Geometry: see drawing. Coordinates: mm, zero at the bounding-box minimum. Give positions to 0.01 mm unless a question says otherwise; leave off trailing zeros. Order: outer loops, then holes, each group sorted by start corner. A loop starts at its lowest first (then second) coordinate and runs counter-clockwise, first axis right, second up. Notation, with made-up numbers: (55, 13) - (96, 13) arc R22 ccw to (96, 43) - close; hole circle Ø5 at (-24.5, 8.5). An arc over 180 degrees is marked (long way). One line per item, written item: value.
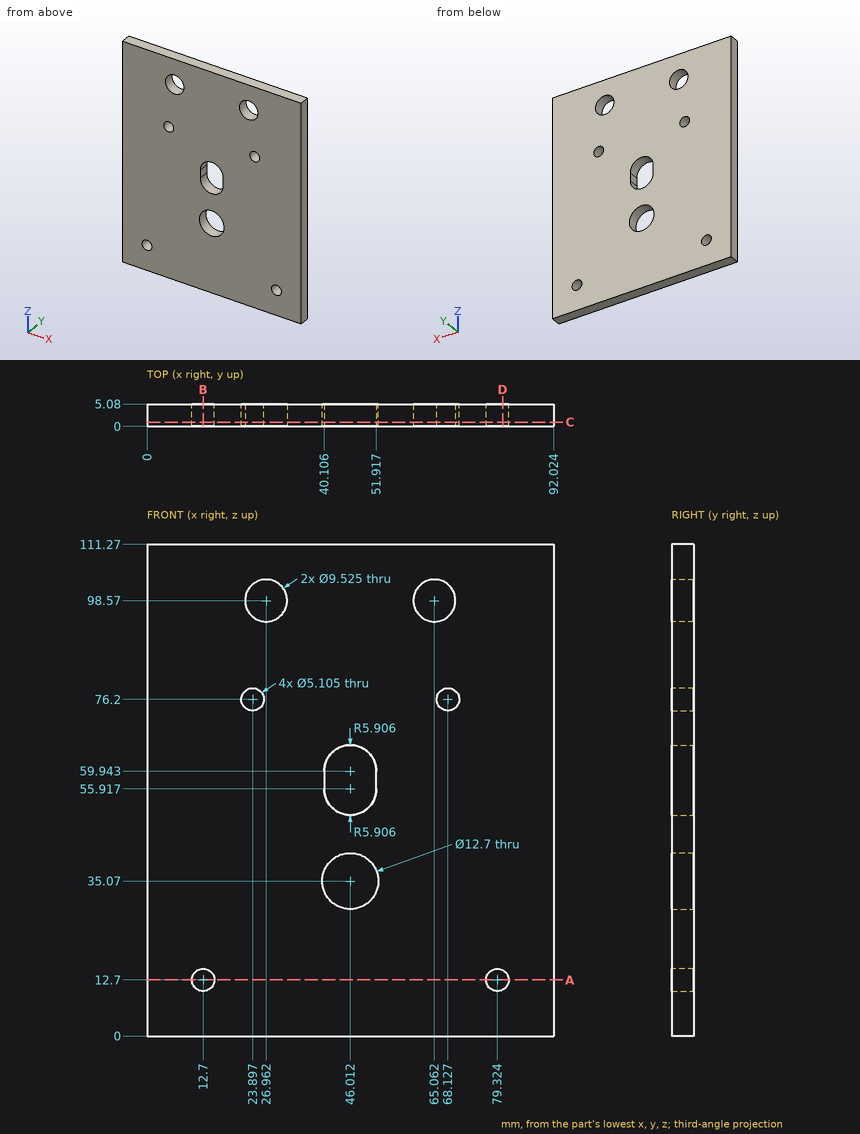
1) Section C-C, the plane y = 0.95. Count the separate pieces of the cut face and the enclosed holes in it, then the cut area to 3 significant figures.
Answers below:
separate pieces: 1
enclosed holes: 8
area: 9,730 mm^2
2) Section D-D, the plane x = 80.5. Return loops of the section in (y, z) (1 decimal), then the cut area to 3 significant figures.
Answers below:
outline: (0, 0) - (5.1, 0) - (5.1, 10.4) - (0, 10.4) - close; (0, 15) - (5.1, 15) - (5.1, 111.3) - (0, 111.3) - close
area: 542 mm^2
3) Section B-B, the plane x = 12.7. Return loops of the section in (y, z).
Answers below:
outline: (0, 0) - (5.08, 0) - (5.08, 10.15) - (0, 10.15) - close; (0, 15.25) - (5.08, 15.25) - (5.08, 111.27) - (0, 111.27) - close
4) Section A-A, the plane z = 12.7. Return loops of the section in (x, y).
Answers below:
outline: (0, 0) - (10.15, 0) - (10.15, 5.08) - (0, 5.08) - close; (15.25, 0) - (76.77, 0) - (76.77, 5.08) - (15.25, 5.08) - close; (81.88, 0) - (92.02, 0) - (92.02, 5.08) - (81.88, 5.08) - close
5) Material intervals for line 1 along X through (y, z) = (1.7, 12.7); line 2 along X through (y, z) = (0.9, 57.5); line 3 along Z through (x, y) = (47, 0.55) (1 decimal), sorted ascending.
Answers below:
line 1: 0 to 10.15, 15.25 to 76.77, 81.88 to 92.02
line 2: 0 to 40.11, 51.92 to 92.02
line 3: 0 to 28.8, 41.3 to 50.1, 65.8 to 111.3
